Check sheet for the modelled part. Datum: model origin and axes. Units: mm. A direction names the side the tool comes from. Give positions to 0.01 mm unless a question says otherwise; leave off trailing zeros. Order: outer loops, then holes, each group sorted by start corner. A loop starts at its lowest first (then second) coordinate and runs counter-clockwise, first axis right, second up. Notation, with made-up numbers: (11.25, 7.5) -> (27.25, 7.5) arc R25 ccw to (27.25, 27.5) -> close; hole circle Ø8 at (86, 34.25). An arc over 180 degrees is marked (long way). One line per question, with ' | ' between items.
```python
from build123d import *

# Parameters (mm, degrees)
CROQUIS1_R                 = 20
CROQUIS1_R_2               = 2
CROQUIS1_R_3               = 3
SALIENTE_EXTRUIR1_DEPTH    = 3
CROQUIS2_R                 = 7.5
CROQUIS2_R_2               = 3
SALIENTE_EXTRUIR2_DEPTH    = 8
CORTAR_EXTRUIR1_DEPTH      = 31.347981811
CORTAR_EXTRUIR1_DEPTH_BACK = 31.347981811
CROQUIS3_R                 = 1.5


with BuildPart() as part:
    # Croquis1 → Saliente-Extruir1 (new body)
    with BuildSketch(Plane(origin=(0, 0, 0), x_dir=(1, 0, 0), z_dir=(0, 1, 0))):
        with Locations(Location((0, 0, 0), (0, 0, 270))):
            Circle(CROQUIS1_R)
        with Locations(Location((0, 14, 0), (0, 0, 270))):
            Circle(CROQUIS1_R_2, mode=Mode.SUBTRACT)
        with Locations(Location((12.124355653, -7, 0), (0, 0, 270))):
            Circle(CROQUIS1_R_2, mode=Mode.SUBTRACT)
        with Locations(Location((-12.124355653, -7, 0), (0, 0, 270))):
            Circle(CROQUIS1_R_2, mode=Mode.SUBTRACT)
        with Locations(Location((0, 0, 0), (0, 0, 270))):
            Circle(CROQUIS1_R_3, mode=Mode.SUBTRACT)
    extrude(amount=SALIENTE_EXTRUIR1_DEPTH)

    # Croquis2 → Saliente-Extruir2 (add)
    with BuildSketch(Plane(origin=(0, 3, 0), x_dir=(1, 0, 0), z_dir=(0, 1, 0))):
        with Locations(Location((0, 0, 0), (0, 0, 270))):
            Circle(CROQUIS2_R)
        with Locations(Location((0, 0, 0), (0, 0, 270))):
            Circle(CROQUIS2_R_2, mode=Mode.SUBTRACT)
    extrude(amount=SALIENTE_EXTRUIR2_DEPTH)

    # Croquis3 → Cortar-Extruir1 (cut, two sides: drawn at the far end of the back side and taken through both)
    with BuildSketch(Plane(origin=(0, 0, 0), x_dir=(0, 0, -1), z_dir=(1, 0, 0)).offset(-CORTAR_EXTRUIR1_DEPTH_BACK)):
        with Locations((0, 7)):
            Circle(CROQUIS3_R)
    extrude(amount=CORTAR_EXTRUIR1_DEPTH + CORTAR_EXTRUIR1_DEPTH_BACK, mode=Mode.SUBTRACT)


solid = part.part
```
Q1. Section check A-A (x = 0). Enter the section's corners in (y, z), and give its area (3 significant figures).
Result sheet:
outline: (0, -20) -> (3, -20) -> (3, -16) -> (0, -16) -> close; (0, -12) -> (3, -12) -> (3, -7.5) -> (11, -7.5) -> (11, -3) -> (0, -3) -> close; (0, 3) -> (11, 3) -> (11, 7.5) -> (3, 7.5) -> (3, 20) -> (0, 20) -> close | area: 162 mm2
Q2. Section check D-D (y = 7.5). Enter the section's corners in (x, z).
Result sheet:
outline: (-7.37, -1.41) arc R7.5 ccw to (7.37, -1.41) -> (2.65, -1.41) arc R3 cw to (-2.65, -1.41) -> close; (-7.37, 1.41) -> (-2.65, 1.41) arc R3 cw to (2.65, 1.41) -> (7.37, 1.41) arc R7.5 ccw to start
Q3. Access from +Z, -Z, +X, -X, +Y, -Y to the whole of each face (thin tool, end or side, straight path). Record for faces 5 (the face through (0, 3, 9)), 6 (the face through (-19.524, 1.479, -4.336)).
Result sheet:
face 5: +Y | face 6: +Y, -Y
Q4. Section check B-B (z = 0). Enter the section's corners in (x, y), and give its area (3 significant figures).
Result sheet:
outline: (-20, 0) -> (-3, 0) -> (-3, 5.5) -> (-7.5, 5.5) -> (-7.5, 3) -> (-20, 3) -> close; (-7.5, 8.5) -> (-3, 8.5) -> (-3, 11) -> (-7.5, 11) -> close; (3, 0) -> (20, 0) -> (20, 3) -> (7.5, 3) -> (7.5, 5.5) -> (3, 5.5) -> close; (3, 8.5) -> (7.5, 8.5) -> (7.5, 11) -> (3, 11) -> close | area: 147 mm2
Q5. Depth check by flat-ended pin: pin 1 Ø1 at (x, z) = (-11.5, -6.5) entering from +Y; pin 2 Ø3 at (y, z) = (8, -2.5) entering from +X; pin 3 Ø3 at (x, z) = (12.12, 7) entering from +Y; pin 4 Ø5 at (y, z) = (7, 0) entering from -X. Enter the tip coordinate at first touch or a pass-through.
Result sheet:
pin 1: stops at y = 3 | pin 2: stops at x = 7.43 | pin 3: passes through | pin 4: stops at x = -7.5
Q6. Mould release check, pull along Z, two halves, no side actions. Record for faces 1 (the face through (-1.2, 1.5, -15.6)), 2 (the face through (-6.654, 6.944, 3.461)), 3 (the face through (0, 0, 4)), 4 (the face through (5.02, 7.07, 1.5)): pulls with the +Z half, pulls with the -Z half, needs draft (parallel to the pull), parting line crosses it, or undercut.
Result sheet:
face 1: undercut | face 2: parting line crosses it | face 3: needs draft | face 4: undercut
Q7. Section check C-C (z = -14). Enter the section's corners in (x, y), and give its area (3 significant figures).
Result sheet:
outline: (-14.28, 0) -> (-2, 0) -> (-2, 3) -> (-14.28, 3) -> close; (2, 0) -> (14.28, 0) -> (14.28, 3) -> (2, 3) -> close | area: 73.7 mm2
Q8. Thickness scan on line 1 (Z direction, x = 1, y = 1.75); line 2 (Y direction, x = 4, z = -9); line 3 (Z direction, x = -4.5, y = 7). Record the ranges inside material, lowest first.
Result sheet:
line 1: z = -19.97 to -15.73, -12.27 to -2.83, 2.83 to 19.97 | line 2: y = 0 to 3 | line 3: z = -6 to -1.5, 1.5 to 6
